Autodesk Inventor part; units mm, degrees
ref_plane "YZ Plane" through (0, 0, 0) normal (1, 0, 0) x (0, 1, 0)
ref_plane "XZ Plane" through (0, 0, 0) normal (0, 1, 0) x (-1, 0, 0)
ref_plane "XY Plane" through (0, 0, 0) normal (0, 0, 1) x (1, 0, 0)
sketch "Sketch1" plane through (0, 0, 0) normal (0, 1, 0) x (-1, 0, 0)
  circle A0 centre (0, 0) radius 22.5
  circle A1 centre (0, 0) radius 33
  circle A2 centre (0, 0) radius 23
  circle A3 centre (0, 0) radius 32.5
  dimension "d0" = 45
  dimension "d1" = 66
  dimension "d2" = 0.5
  dimension "d3" = 0.5
extrude "Extrusion1" add sketch "Sketch1" along normal mid plane 14 contours A1 | A2 | A3
extrude "Extrusion2" cut sketch "Sketch1" along normal mid plane 7
properties part number "Thrust Bearing 51109 - 45x66x14mm" material "Stainless Steel"
Build history of the part. All positions in model axes, mm. A direction names the side the tool comes from. Give positions to 0.01 mm unless a question says otherwise; leave off trailing zeros. Loops run counter-clockwise (first coordinate to the right, second up) from the corner with the lowest first, then second, coordinate; pieces in that order, holes last. Notation, with made-up numbers: (12.25, 74) - (61.25, 74) arc R15 ccw to (61.25, 90) - close; hole circle Ø6 at (41, -21). An arc over 180 degrees is marked (long way). Use a Markdown table: item, result.
(1) Band-saw the part on D-D (z = -26.5). Give the cut face in (x, y).
Taken from the geometry:
| item | result |
|---|---|
| outline | (-19.67, -7) - (19.67, -7) - (19.67, -3.5) - (18.81, -3.5) - (18.81, 3.5) - (19.67, 3.5) - (19.67, 7) - (-19.67, 7) - (-19.67, 3.5) - (-18.81, 3.5) - (-18.81, -3.5) - (-19.67, -3.5) - close |
(2) Band-saw the part on C-C (y = -5.75). Give the cut face in (x, z), and give its area (3 significant figures).
Taken from the geometry:
| item | result |
|---|---|
| outline | circle Ø66 at (0, 0); hole circle Ø45 at (0, 0) |
| area | 1,830 mm2 |
(3) Pull direction X, two halves, no side cores. Call faces 1 (the face through (-10.382, -5.226, -19.961)), 2 (the face through (-24.29, 3.5, -21.85)), 3 (the face through (-31, 0.05, 9.76)), 4 (the face through (-17, 3.5, -15)): +X half, -X half, draft (parallel to the pull), parting line (faces both ways), or undercut.
Taken from the geometry:
| item | result |
|---|---|
| face 1 | undercut |
| face 2 | draft |
| face 3 | parting line |
| face 4 | undercut |
(4) Which spindle directions (+Z, -Z, +X, -X, +Y, -Y) get a long thin tool onto all of the face, cutting with end or side? Do faces 5 (the face through (-30.5, -5.2, -12.6)), 6 (the face through (-17, -3.5, -15)). Say none if no direction does.
Taken from the geometry:
| item | result |
|---|---|
| face 5 | +Y, -Y |
| face 6 | none |
(5) Drop flat-ended pins along their axis: pin 1 Ø4 at (y, z) = (3, -21) entering from -X; pin 2 Ø23 at (x, z) = (-1, -10) entering from -Y; pin 3 Ø3 at (x, y) = (-16, 3) entering from -Z; pin 4 Ø3 at (y, z) = (5.5, 11) entering from -X. Give the stop position or say it passes through.
Taken from the geometry:
| item | result |
|---|---|
| pin 1 | x = -26.94 |
| pin 2 | through |
| pin 3 | z = -29.6 |
| pin 4 | x = -31.6 |
(6) Wall check: line 1 along Z through (x, y) = (0, 1.5); line 2 along Y through (x, z) = (-10.5, -20); line 3 along X through (y, z) = (1.75, -20.5). Give the ranges that are in metal, low to high.
Taken from the geometry:
| item | result |
|---|---|
| line 1 | -32.5 to -23, 23 to 32.5 |
| line 2 | -7 to -3.5, 3.5 to 7 |
| line 3 | -25.22 to -10.43, 10.43 to 25.22 |
(7) Band-saw the part on A-A (x = 0). Give the cut face in (y, z).
Taken from the geometry:
| item | result |
|---|---|
| outline | (-7, -33) - (-3.5, -33) - (-3.5, -32.5) - (3.5, -32.5) - (3.5, -33) - (7, -33) - (7, -22.5) - (3.5, -22.5) - (3.5, -23) - (-3.5, -23) - (-3.5, -22.5) - (-7, -22.5) - close; (-7, 22.5) - (-3.5, 22.5) - (-3.5, 23) - (3.5, 23) - (3.5, 22.5) - (7, 22.5) - (7, 33) - (3.5, 33) - (3.5, 32.5) - (-3.5, 32.5) - (-3.5, 33) - (-7, 33) - close |
(8) Band-saw the part on B-B (z = 0). Give the cut face in (x, y).
Taken from the geometry:
| item | result |
|---|---|
| outline | (-33, -7) - (-22.5, -7) - (-22.5, -3.5) - (-23, -3.5) - (-23, 3.5) - (-22.5, 3.5) - (-22.5, 7) - (-33, 7) - (-33, 3.5) - (-32.5, 3.5) - (-32.5, -3.5) - (-33, -3.5) - close; (22.5, -7) - (33, -7) - (33, -3.5) - (32.5, -3.5) - (32.5, 3.5) - (33, 3.5) - (33, 7) - (22.5, 7) - (22.5, 3.5) - (23, 3.5) - (23, -3.5) - (22.5, -3.5) - close |
